from build123d import *

# Parameters (mm, degrees)
SKETCH1_W           = 101.6
SKETCH1_H           = 25.4
SKETCH1_R           = 3.429
BOSS_EXTRUDE1_DEPTH = 6.35


with BuildPart() as part:
    # Sketch1 → Boss-Extrude1 (new body)
    with BuildSketch(Plane.XY):
        Rectangle(SKETCH1_W, SKETCH1_H)
        Circle(SKETCH1_R, mode=Mode.SUBTRACT)
        with Locations((-38.1, 0)):
            Circle(SKETCH1_R, mode=Mode.SUBTRACT)
        with Locations(Location((38.1, 0, 0), (0, 0, 180))):
            Circle(SKETCH1_R, mode=Mode.SUBTRACT)
    extrude(amount=BOSS_EXTRUDE1_DEPTH)


solid = part.part
Model file for the job. Use its own axes, mm. Round coordinates to 2 decimals unless told otherwise and drop trailing zeros. Loops run counter-clockwise (first coordinate to the right, second up) from the corner with the lowest first, then second, coordinate; pieces in that order, holes last. Notation, with made-up numbers: M 14.25,5.5 L 70.25,5.5 A20 ccw 70.25,35.5 Z; hole C -18.75,-23 d4. An arc over 180 degrees is marked long. One line per question, with ' | ' between items.
1) Drill centre lines: line 1 along Y through (x, z) = (38.1, 1.75); line 2 along Y through (x, z) = (39.5, 5.25); line 3 along X through (y, z) = (1.75, 0.5). Where is each one in solid material? Low to high.
Solved:
line 1: y = -12.7 to -3.43, 3.43 to 12.7 | line 2: y = -12.7 to -3.13, 3.13 to 12.7 | line 3: x = -50.8 to -41.05, -35.15 to -2.95, 2.95 to 35.15, 41.05 to 50.8
2) Flat gauge pin, fed straight in: pin 1 (11 mm diameter, centred on x = -38.1, y = 0, fed in from +Z). Where does the tip first touch, or does it go through?
Solved:
pin 1: stops at z = 6.35
3) Band-saw the part on B-B (z = 5). Give the cut face in (x, y), then the cut area to 3 significant figures.
Solved:
outline: M -50.8,-12.7 L 50.8,-12.7 L 50.8,12.7 L -50.8,12.7 Z; hole C -38.1,0 d6.86; hole C 0,0 d6.86; hole C 38.1,0 d6.86 | area: 2,470 mm²
4) Mould opens along Y. For faces 1 (the flat face through (-1, -12.7, 3)), 2 (the cylindrical face through (-40.627, 2.317, 3.131)), 3 (the flat face through (-1, -5, 0)) say: +Y half, -Y half, draft (parallel to the pull), parting line (faces both ways), or undercut.
Solved:
face 1: -Y half | face 2: undercut | face 3: draft
5) Band-saw the part on C-C (x = -38.1). Give the cut face in (y, z).
Solved:
outline: M -12.7,0 L -3.43,0 L -3.43,6.35 L -12.7,6.35 Z; M 3.43,0 L 12.7,0 L 12.7,6.35 L 3.43,6.35 Z
6) Band-saw the part on A-A (y = 0). Give the cut face in (x, z).
Solved:
outline: M -50.8,0 L -41.53,0 L -41.53,6.35 L -50.8,6.35 Z; M -34.67,0 L -3.43,0 L -3.43,6.35 L -34.67,6.35 Z; M 3.43,0 L 34.67,0 L 34.67,6.35 L 3.43,6.35 Z; M 41.53,0 L 50.8,0 L 50.8,6.35 L 41.53,6.35 Z
